from build123d import *

# Parameters (mm, degrees)
MBODY_DEPTH             = 40
SKETCH5_R               = 0.75
FRONTSCREWS_DEPTH       = 3
SKETCH7_R               = 2.75
GUIDKNOB_DEPTH          = 4
SERVOCUT_DEPTH          = 40.5
ROUNDEDGE_R             = 20
SKETCH23_W              = 70
SKETCH23_H              = 40
TOPPUSHDOWN_DEPTH       = 9
SKETCH12_R              = 2
SERVOHOLDERS_DEPTH      = 2.25
SKETCH24_R              = 0.75
SERVOHOLDERSCREWS_DEPTH = 3.25
SKETCH14_W              = 30
SKETCH14_H              = 40
CABLEACCESS_DEPTH       = 20.25
ROUNDEDGES_R            = 1
SKETCH8_R               = 0.75
SIDESCREWS1_DEPTH       = 3
SIDESCREWS2_START       = 3
SKETCH17_R              = 0.75
SIDESCREWS2_DEPTH       = 3
SKETCH18_R              = 3.75
SIDEGUIDEHOLE_DEPTH     = 40.5


with BuildPart() as part:
    # Sketch4 → MBODY (new body)
    with BuildSketch(Plane(origin=(0, 0, 0), x_dir=(1, 0, 0), z_dir=(0, 1, 0))):
        Polygon((-5, 20), (-25.25, 20), (-25.25, -75), (-5, -75), (15.25, -75), (15.25, 20), align=None)
    extrude(amount=MBODY_DEPTH)

    # Sketch5 → FrontScrews (cut)
    with BuildSketch(Plane(origin=(0, 0, -20), x_dir=(-1, 0, 0), z_dir=(0, 0, -1))):
        with Locations((0, 5)):
            Circle(SKETCH5_R)
        with Locations((10, 5)):
            Circle(SKETCH5_R)
        with Locations((10, 15)):
            Circle(SKETCH5_R)
        with Locations((0, 15)):
            Circle(SKETCH5_R)
        with Locations((0, 25)):
            Circle(SKETCH5_R)
        with Locations((10, 25)):
            Circle(SKETCH5_R)
        with Locations((10, 35)):
            Circle(SKETCH5_R)
        with Locations((0, 35)):
            Circle(SKETCH5_R)
    extrude(amount=-FRONTSCREWS_DEPTH, mode=Mode.SUBTRACT)

    # Sketch7 → GUIDKNOB (add)
    with BuildSketch(Plane(origin=(0, 0, -20), x_dir=(-1, 0, 0), z_dir=(0, 0, -1))):
        with Locations((5, 20)):
            Circle(SKETCH7_R)
    extrude(amount=GUIDKNOB_DEPTH)

    # Sketch10 → ServoCut (cut)
    with BuildSketch(Plane(origin=(15.25, 0, 0), x_dir=(0, 0, -1), z_dir=(1, 0, 0))):
        Polygon((-65.5, 20), (-65.5, 30.5), (-24.5, 30.5), (-24.5, 9.5), (-65.5, 9.5), align=None)
    extrude(amount=-SERVOCUT_DEPTH, mode=Mode.SUBTRACT)

    # RoundEdge
    roundedge_edges = [part.edges().sort_by_distance(p)[0] for p in [
        (-5, 0, 75),
        (-5, 40, 75),
    ]]
    fillet(roundedge_edges, radius=ROUNDEDGE_R - 0.0001)  # a hair under: the kernel refuses the full size

    # Sketch23 → TOPPUSHDOWN (cut)
    with BuildSketch(Plane(origin=(15.25, 0, 0), x_dir=(0, 0, -1), z_dir=(1, 0, 0))):
        with Locations((-44.894780196, 20)):
            Rectangle(SKETCH23_W, SKETCH23_H)
    extrude(amount=-TOPPUSHDOWN_DEPTH, mode=Mode.SUBTRACT)

    # Sketch12 → SERVOHOLDERS (add)
    with BuildSketch(Plane(origin=(6.25, 0, 0), x_dir=(0, 0, -1), z_dir=(1, 0, 0))):
        with Locations(Location((-69.75, 25, 0), (0, 0, 180))):
            Circle(SKETCH12_R)
        with Locations(Location((-69.75, 15, 0), (0, 0, 180))):
            Circle(SKETCH12_R)
        with Locations(Location((-20.25, 15, 0), (0, 0, 180))):
            Circle(SKETCH12_R)
        with Locations(Location((-20.25, 25, 0), (0, 0, 180))):
            Circle(SKETCH12_R)
    extrude(amount=SERVOHOLDERS_DEPTH)

    # Sketch24 → SERVOHOLDERSCREWS (cut)
    with BuildSketch(Plane(origin=(8.5, 0, 0), x_dir=(0, 0, -1), z_dir=(1, 0, 0))):
        with Locations((-69.75, 25)):
            Circle(SKETCH24_R)
        with Locations((-69.75, 15)):
            Circle(SKETCH24_R)
        with Locations((-20.25, 25)):
            Circle(SKETCH24_R)
        with Locations((-20.25, 15)):
            Circle(SKETCH24_R)
    extrude(amount=-SERVOHOLDERSCREWS_DEPTH, mode=Mode.SUBTRACT)

    # Sketch14 → CABLEACCESS (cut)
    with BuildSketch(Plane.ZY.offset(25.25)):
        with Locations((60, 20)):
            Rectangle(SKETCH14_W, SKETCH14_H)
    extrude(amount=-CABLEACCESS_DEPTH, mode=Mode.SUBTRACT)

    # ROUNDEDGES
    roundedges_edges = [part.edges().sort_by_distance(p)[0] for p in [
        (6.25, 9.5, 45),
        (6.25, 20, 24.5),
        (15.25, 20, 9.894780196),
        (-25.25, 20, -20),
        (15.25, 20, -20),
        (-5, 5.857835087, 69.142164913),
        (-25.25, 9.5, 34.75),
        (-15.125, 9.5, 45),
        (-25.25, 30.5, 34.75),
        (-15.125, 30.5, 45),
        (-5, 4.75, 45),
        (-15.125, 0, 45),
        (-5, 40, 50.00005),
        (-15.125, 40, 45),
        (-5, 30.5, 55.25),
        (-5, 20, 65.5),
        (-5, 34.142164913, 69.142164913),
        (-5, 35.25, 45),
        (-5, 0, 50.00005),
        (-5, 9.5, 55.25),
        (-25.25, 35.25, 45),
        (15.25, 40, -5.052609902),
        (-25.25, 4.75, 45),
        (-5, 40, -20),
        (-25.25, 40, 12.5),
        (-25.25, 20, 24.5),
        (-5, 0, -20),
        (15.25, 0, -5.052609902),
        (-25.25, 0, 12.5),
        (6.25, 5.857835087, 69.142164913),
        (6.25, 40, 32.447440098),
        (6.25, 0, 32.447440098),
        (10.75, 0, 9.894780196),
        (6.25, 20, 65.5),
        (6.25, 30.5, 45),
        (6.25, 34.142164913, 69.142164913),
        (6.25, 20, 9.894780196),
        (10.75, 40, 9.894780196),
    ]]
    fillet(roundedges_edges, radius=ROUNDEDGES_R)

    # Sketch8 → SideScrews1 (cut)
    with BuildSketch(Plane(origin=(15.25, 50, 0), x_dir=(0, 0, -1), z_dir=(-1, 0, 0))):
        with Locations(Location((14, 37, 0), (0, 0, 180))):
            Circle(SKETCH8_R)
        with Locations(Location((14, 30, 0), (0, 0, 180))):
            Circle(SKETCH8_R)
        with Locations(Location((7, 37, 0), (0, 0, 180))):
            Circle(SKETCH8_R)
        with Locations(Location((14, 23, 0), (0, 0, 180))):
            Circle(SKETCH8_R)
        with Locations(Location((0, 37, 0), (0, 0, 180))):
            Circle(SKETCH8_R)
        with Locations(Location((7, 23, 0), (0, 0, 180))):
            Circle(SKETCH8_R)
        with Locations(Location((0, 30, 0), (0, 0, 180))):
            Circle(SKETCH8_R)
        with Locations(Location((0, 23, 0), (0, 0, 180))):
            Circle(SKETCH8_R)
    extrude(amount=SIDESCREWS1_DEPTH, mode=Mode.SUBTRACT)

    # Sketch17 → SideScrews2 (cut)
    with BuildSketch(Plane(origin=(-25.25, 15, 0), x_dir=(0, -1, 0), z_dir=(1, 0, 0)).offset(SIDESCREWS2_START)):
        with Locations(Location((-12, 14, 0), (0, 0, 270))):
            Circle(SKETCH17_R)
        with Locations(Location((-5, 14, 0), (0, 0, 270))):
            Circle(SKETCH17_R)
        with Locations(Location((2, 14, 0), (0, 0, 270))):
            Circle(SKETCH17_R)
        with Locations(Location((2, 7, 0), (0, 0, 270))):
            Circle(SKETCH17_R)
        with Locations(Location((-12, 7, 0), (0, 0, 270))):
            Circle(SKETCH17_R)
        with Locations(Location((-12, -0.00489205, 0), (0, 0, 90))):
            Circle(SKETCH17_R)
        with Locations(Location((-5, -0.00489205, 0), (0, 0, 90))):
            Circle(SKETCH17_R)
        with Locations(Location((2, -0.00489205, 0), (0, 0, 90))):
            Circle(SKETCH17_R)
    extrude(amount=-SIDESCREWS2_DEPTH, mode=Mode.SUBTRACT)

    # Sketch18 → SIDEGUIDEHOLE (cut)
    with BuildSketch(Plane(origin=(-25.25, 25, 0), x_dir=(0, 1, 0), z_dir=(1, 0, 0))):
        with Locations(Location((-5, -7, 0), (0, 0, 270))):
            Circle(SKETCH18_R)
    extrude(amount=SIDEGUIDEHOLE_DEPTH, mode=Mode.SUBTRACT)


solid = part.part
Model file for the job. Use its own axes, mm. A direction names the side the tool comes from. Give positions to 0.01 mm unless a question says otherwise; leave off trailing zeros. Loops run counter-clockwise (first coordinate to the right, second up) from the corner with the lowest first, then second, coordinate; pieces in that order, holes last. Notation, with made-up numbers: (62.25, 55) -> (80.25, 55) arc R14 ccw to (80.25, 65) -> close; hole circle Ø5 at (26.5, 42). An arc over 180 degrees is marked (long way). Use a Markdown table: item, result. Add a question column.
(1) Slice it at B-B on x = -12.5. List the corners of the cut face in (y, z).
(2) Drop flat-ended pins along their axis: pin 1 Ø1.4 at (y, z) = (13, -7) entering from -X; pin 2 Ø6.5 at (x, y) = (-3, 16) entering from +Z; pin 3 Ø1.2 at (y, z) = (14, 70) entering from +X. Give the stop position or say it passes through.
(3) Tool access for faces 1 (the flat face through (-9, 20, 24.5)), 2 (the cylindrical face through (7.359, 26.217, 18.663)), 3 (the flat face through (8.5, 16, 20)), 4 (the flat face through (-5, 20, 69)): list every direction of +Z, -Z, +X, -X, +Y, -Y with a clear straight run to the whole face (end or side of a thin tool).
(4) Wall check: line 1 along Y through (x, z) = (0, -18); line 2 along Y through (x, z) = (7.85, 69.75); line 3 along Y through (x, z) = (14.35, -14). Give the ranges that are in metal, low to high.
(5) Slice it at C-C on z = 15.5. List the corners of the cut face in (x, y).
(6) Mould opens along Z. For faces 5 (the flat face through (1, 20, 65.5)), 6 (the flat face through (8.5, 16, 70)), 7 (the flat face through (-15, 5, 45)) say: +Z half, -Z half, draft (parallel to the pull), parting line (faces both ways), or undercut.
(7) Slice it at A-A on z = 28. List the corners of the cut face in (x, y).
Filled sheet:
| question | item | result |
|---|---|---|
| 1 | outline | (0, -19) arc R1 ccw to (1, -20) -> (39, -20) arc R1 ccw to (40, -19) -> (40, 44) arc R1 ccw to (39, 45) -> (31.5, 45) arc R1 ccw to (30.5, 44) -> (30.5, 24.5) -> (9.5, 24.5) -> (9.5, 44) arc R1 ccw to (8.5, 45) -> (1, 45) arc R1 ccw to (0, 44) -> close; hole circle Ø7.5 at (20, -7) |
| 2 | pin 1 | x = -22.25 |
| 2 | pin 2 | z = 74.99 |
| 2 | pin 3 | x = 8.5 |
| 3 | face 1 | +X, -X |
| 3 | face 2 | +X |
| 3 | face 3 | +Z, +X, +Y, -Y |
| 3 | face 4 | +Z, -X, +Y, -Y |
| 4 | line 1 | 0 to 4.25, 5.75 to 14.25, 15.75 to 24.25, 25.75 to 34.25, 35.75 to 40 |
| 4 | line 2 | 13 to 14.25, 15.75 to 17, 23 to 24.25, 25.75 to 27 |
| 4 | line 3 | 0.01 to 12.25, 13.75 to 19.25, 20.75 to 26.25, 27.75 to 39.99 |
| 5 | outline | (-25.25, 1) arc R1 ccw to (-24.25, 0) -> (5.25, 0) arc R1 ccw to (6.25, 1) -> (6.25, 39) arc R1 ccw to (5.25, 40) -> (-24.25, 40) arc R1 ccw to (-25.25, 39) -> close |
| 6 | face 5 | undercut |
| 6 | face 6 | draft |
| 6 | face 7 | +Z half |
| 7 | outline | (-25.25, 1) arc R1 ccw to (-24.25, 0) -> (5.25, 0) arc R1 ccw to (6.25, 1) -> (6.25, 8.5) arc R1 ccw to (5.25, 9.5) -> (-24.25, 9.5) arc R1 ccw to (-25.25, 8.5) -> close; (-25.25, 31.5) arc R1 ccw to (-24.25, 30.5) -> (5.25, 30.5) arc R1 ccw to (6.25, 31.5) -> (6.25, 39) arc R1 ccw to (5.25, 40) -> (-24.25, 40) arc R1 ccw to (-25.25, 39) -> close |
